Geometry check sheet. Reference: the model listing, model coordinates, mm. Face numbers are marked on the shaded views. A direction names the side the tool comes from. Round coordinates to 2 decimals unless told otherwise and drop trailing zeros. Order: outer loops, then holes, each group sorted by start corner. A loop starts at its lowest first (then second) coordinate and runs counter-clockwise, first axis right, second up.
(1) Cross-section at D-D on y = -6.5. Enter the section's corners in (x, z), and give its area (3 significant figures).
(2) Gauge pin test, flat ends, axial feed: P1, Ø0.9, axis at x = -1, z = 1.5, coming from the -Y side; P2, Ø0.9, axis at x = -0.5, z = 1.5, coming from the +Y side; P3, Ø6, axis at x = -0.5, y = -3, coming from the +Z side; P4, Ø3, axis at y = -6.5, z = 1.5, coming from the +X side. Record the tip position at first contact, or that the pin passes through.
(3) Draft check along X on the marked faces 5, 6, 7 and 8. Enter one of: pulls with the +X half, pulls with the -X half, needs draft (parallel to the pull), parting line crosses it, or undercut.
(4) Set-up check for the marked faces 1, 2, 3 and 4: record each of +Z, -Z, +X, -X, +Y, -Y from which the full face is reachable in a straight line by a thin tool's end or side.
(5) Cross-section at A-A on z = 5. Enter the section's corners in (x, y), and give its area (3 significant figures).
(6) Cross-section at C-C on y = -4. Enter the section's corners in (x, z).
(7) Thickness scan on L1, parallel to Y at x = 15.25, z = 0.4; L2, parallel to Y at x = 15, z = 4.25; L3, parallel to X at y = 1.75, z = 0.75. Record the ranges inside material, lowest first.
(8) Cross-section at B-B on z = 2.5. Enter the section's corners in (x, y).
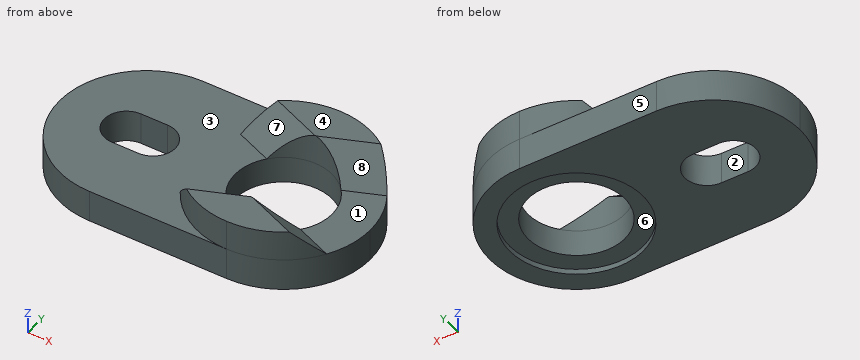
from build123d import *

# Parameters (mm, degrees)
F0_R        = 5.45
F1_DEPTH    = 3.6
F3_DEPTH    = 3.4
F4_T4_DEPTH = 30.0168298797
F5_T4_DEPTH = 28.3957620677
F6_T4_DEPTH = 30.0168298797
F7_T4_DEPTH = 28.3957620678
F8_R        = 7.5
F9_DEPTH    = 0.6


# Not quite as in the source:
# - a fillet or chamfer that OpenCascade refuses, or shapes differently, is made with other operations: its cross-section is extruded or revolved along the edge and cut away or added


with BuildPart() as f1:
    # F0 (on Top) → F1 (new body)
    with BuildSketch(Plane.XY):
        with BuildLine():
            Line((15.25, 9.75), (-0.25, 9.75))
            ThreePointArc((-0.25, 9.75), (-7.1442911166, 6.8942911166), (-10, 0))
            ThreePointArc((-10, 0), (-7.1442911166, -6.8942911166), (-0.25, -9.75))
            Line((-0.25, -9.75), (15.25, -9.75))
            ThreePointArc((15.25, -9.75), (22.1442911166, -6.8942911166), (25, 0))
            ThreePointArc((25, 0), (22.1442911166, 6.8942911166), (15.25, 9.75))
        make_face()
        with BuildLine():
            ThreePointArc((-2.5, -2.5), (-5, 0), (-2.5, 2.5))
            Line((-2.5, 2.5), (0.5, 2.5))
            ThreePointArc((0.5, 2.5), (3, 0), (0.5, -2.5))
            Line((0.5, -2.5), (-2.5, -2.5))
        make_face(mode=Mode.SUBTRACT)
        with Locations((15.25, 0)):
            Circle(F0_R, mode=Mode.SUBTRACT)
    extrude(amount=F1_DEPTH)

    # F2 (on face) → F3 (join)
    with BuildSketch(Plane.XY.offset(3.6)):
        with BuildLine():
            Line((6.242174558, 3.7311634656), (10.2148565478, 2.0856247064))
            ThreePointArc((10.2148565478, 2.0856247064), (15.25, 5.45), (20.2851434522, 2.0856247064))
            Line((20.2851434522, 2.0856247064), (24.257825442, 3.7311634656))
            ThreePointArc((24.257825442, 3.7311634656), (20.6668097719, 8.1068287199), (15.25, 9.75))
            ThreePointArc((15.25, 9.75), (9.8331902281, 8.1068287199), (6.242174558, 3.7311634656))
        make_face()
        with BuildLine():
            ThreePointArc((20.2851434522, -2.0856247064), (15.25, -5.45), (10.2148565478, -2.0856247064))
            Line((10.2148565478, -2.0856247064), (6.242174558, -3.7311634656))
            ThreePointArc((6.242174558, -3.7311634656), (9.8331902281, -8.1068287199), (15.25, -9.75))
            ThreePointArc((15.25, -9.75), (20.6668097719, -8.1068287199), (24.257825442, -3.7311634656))
            Line((24.257825442, -3.7311634656), (20.2851434522, -2.0856247064))
        make_face()
    extrude(amount=F3_DEPTH)

    # F4: chamfer of 5 on 1 edges, made by hand


with BuildPart() as f4_tool2:
    # F4_s3 → F4_t4 (new body)
    with BuildSketch(Plane(origin=(-7.8707626189, 3.260176623, 0), x_dir=(0, 0, 1), z_dir=(0.9238795325, -0.3826834324, 0))):
        Polygon((2, -5.8359223436), (7, -10.8359223436), (7, -5.8359223436), align=None)
    extrude(amount=F4_T4_DEPTH)

    split(bisect_by=Plane.XY.offset(3.6), keep=Keep.TOP)


with BuildPart() as f1_1:
    add(f1.part)

    # F4_t1: cut F4_tool2
    add(f4_tool2.part, mode=Mode.SUBTRACT)

    # F5: chamfer of 5 on 1 edges, made by hand


with BuildPart() as f5_tool2:
    # F5_s3 → F5_t4 (new body)
    with BuildSketch(Plane(origin=(7.6698776475, 3.1769673433, 0), x_dir=(0, 0, 1), z_dir=(0.9238795325, 0.3826834324, 0))):
        Polygon((2, 5.8359223436), (7, 0.8359223436), (7, 5.8359223436), align=None)
    extrude(amount=F5_T4_DEPTH)

    split(bisect_by=Plane.XY.offset(3.6), keep=Keep.TOP)


with BuildPart() as f1_2:
    add(f1_1.part)

    # F5_t1: cut F5_tool2
    add(f5_tool2.part, mode=Mode.SUBTRACT)

    # F6: chamfer of 5 on 1 edges, made by hand


with BuildPart() as f6_tool2:
    # F6_s3 → F6_t4 (new body)
    with BuildSketch(Plane(origin=(6.1722062753, -2.556611549, 0), x_dir=(0, 0, 1), z_dir=(0.9238795325, -0.3826834324, 0))):
        Polygon((2, -5.8359223436), (7, -0.8359223436), (7, -5.8359223436), align=None)
    extrude(amount=F6_T4_DEPTH)

    split(bisect_by=Plane.XY.offset(3.6), keep=Keep.TOP)


with BuildPart() as f1_3:
    add(f1_2.part)

    # F6_t1: cut F6_tool2
    add(f6_tool2.part, mode=Mode.SUBTRACT)

    # F7: chamfer of 5 on 1 edges, made by hand


with BuildPart() as f7_tool2:
    # F7_s3 → F7_t4 (new body)
    with BuildSketch(Plane(origin=(18.3635007657, 7.6064110698, 0), x_dir=(0, 0, 1), z_dir=(-0.9238795325, -0.3826834324, 0))):
        Polygon((7, -10.8359223436), (2, -5.8359223436), (7, -5.8359223436), align=None)
    extrude(amount=F7_T4_DEPTH)

    split(bisect_by=Plane.XY.offset(3.6), keep=Keep.TOP)


with BuildPart() as f1_4:
    add(f1_3.part)

    # F7_t1: cut F7_tool2
    add(f7_tool2.part, mode=Mode.SUBTRACT)

    # F8 (on face) → F9 (cut)
    with BuildSketch(Plane(origin=(0, 0, 0), x_dir=(1, 0, 0), z_dir=(0, 0, -1))):
        with Locations((15.25, 0)):
            Circle(F8_R)
    extrude(amount=-F9_DEPTH, mode=Mode.SUBTRACT)


solid = f1_4.part
Found:
1. outline: (-7.52, 0) - (11.51, 0) - (11.51, 0.6) - (18.99, 0.6) - (18.99, 0) - (22.52, 0) - (22.52, 5.22) - (17.88, 7) - (12.62, 7) - (7.98, 5.22) - (7.98, 3.6) - (-7.52, 3.6) - close
1. area: 145 mm2
2. P1: stops at y = -9.75
2. P2: stops at y = 9.75
2. P3: stops at z = 3.6
2. P4: stops at x = 23.62
3. face 5: needs draft
3. face 6: undercut
3. face 7: pulls with the -X half
3. face 8: pulls with the +X half
4. face 1: +Z, +X
4. face 2: +Z, -Z
4. face 3: +Z, -X
4. face 4: +Z, +X, -X, +Y, -Y
5. outline: (7.83, -6.32) arc R9.75 ccw to (22.67, -6.32) - (18.31, -4.51) arc R5.45 cw to (12.19, -4.51) - close; (7.83, 6.32) - (12.19, 4.51) arc R5.45 cw to (18.31, 4.51) - (22.67, 6.32) arc R9.75 ccw to start
5. area: 101 mm2
6. outline: (-9.14, 0) - (8.91, 0) - (8.91, 0.6) - (11.55, 0.6) - (11.55, 4.28) - (9.77, 3.6) - (-9.14, 3.6) - close; (18.95, 0.6) - (21.59, 0.6) - (21.59, 0) - (24.14, 0) - (24.14, 3.6) - (20.73, 3.6) - (18.95, 4.28) - close
7. L1: y = -9.75 to -7.5, 7.5 to 9.75
7. L2: y = -9.75 to -5.44, 5.44 to 9.75
7. L3: x = -9.84 to -4.29, 2.29 to 10.09, 20.41 to 24.84
8. outline: (-0.25, -9.75) - (15.25, -9.75) arc R9.75 ccw to (15.25, 9.75) - (-0.25, 9.75) arc R9.75 ccw to start; hole (-2.5, -2.5) - (0.5, -2.5) arc R2.5 ccw to (0.5, 2.5) - (-2.5, 2.5) arc R2.5 ccw to start; hole circle Ø10.9 at (15.25, 0)
